Autodesk Inventor part; units mm, degrees
ref_plane "YZ Plane" through (0, 0, 0) normal (1, 0, 0) x (0, 1, 0)
ref_plane "XZ Plane" through (0, 0, 0) normal (0, 1, 0) x (-1, 0, 0)
ref_plane "XY Plane" through (0, 0, 0) normal (0, 0, 1) x (1, 0, 0)
sketch "Sketch1" plane through (0, 0, 0) normal (0, 0, 1) x (1, 0, 0)
  line L0 (0, 0) -> (125, 0)
  line L1 (125, 0) -> (125, 50)
  line L2 (125, 50) -> (0, 50)
  line L3 (0, 50) -> (0, 0)
  dimension "d0" = 125
  dimension "d1" = 50
extrude "Extrusion1" add sketch "Sketch1" along normal blind 6.731
sketch "Sketch4" plane through (0, 0, 0) normal (0, 0, -1) x (-1, 0, 0)
  line L0 (-125, 50) -> (0, 50)
  line L1 (-125, 0) -> (-125, 50)
  line L2 (-125, 4.3708) -> (-86.0388, 50)
  line L3 (-112.0129, 19.5805) -> (-106.8941, 15.2097)
  line L4 (-106.8941, 15.2097) -> (-93.907, 30.4195)
  line L5 (-93.907, 30.4195) -> (-99.0259, 34.7903)
  line L6 (0, 0) -> (-125, 0)
  line L7 (-125, 4.3708) -> (-119.8812, 0)
  circle A0 centre (-114.3237, 11.6915) radius 1.588
  dimension "d25" = 6.731
  dimension "d26" = 20
  dimension "d27" = 20
  dimension "d28" = 6.731
  dimension "d29" = 3.176
  dimension "d30" = 3.3655
  dimension "d31" = 7.5
  dimension "d40" = 60
extrude "LCD_Cut" cut sketch "Sketch4" against normal up to next contours L0 L2 L1 | L5 L4 L3 L2 | A0
sketch "Sketch2" plane through (0, 0, 6.731) normal (0, 0, 1) x (1, 0, 0)
  line L0 (0, 0) -> (125, 0)
  line L1 (125, 0) -> (125, 50)
  line L2 (0, 50) -> (0, 0)
  line L3 (20, 0) -> (40, 0)
  line L4 (40, 0) -> (40, -6.731)
  line L5 (40, -6.731) -> (20, -6.731)
  line L6 (20, -6.731) -> (20, 0)
  line L7 (105, 0) -> (85, 0)
  line L8 (85, 0) -> (85, -6.731)
  line L9 (85, -6.731) -> (105, -6.731)
  line L10 (105, -6.731) -> (105, 0)
  line L11 (0, 35) -> (-6.731, 35)
  line L12 (-6.731, 35) -> (-6.731, 15)
  line L13 (-6.731, 15) -> (0, 15)
  line L14 (0, 15) -> (0, 35)
  line L15 (86.0388, 50) -> (0, 50)
  line L16 (20, 50) -> (40, 50)
  line L17 (40, 50) -> (40, 56.731)
  line L18 (40, 56.731) -> (20, 56.731)
  line L19 (20, 56.731) -> (20, 50)
  point P0 (-6.731, 25)
  point P1 (0, 25)
  dimension "d4" = 6.731
  dimension "d5" = 20
  dimension "d6" = 20
  dimension "d7" = 20
extrude "Tabs Pos" add sketch "Sketch2" against normal blind 6.731
sketch "Sketch3" plane through (0, 0, 0) normal (0, 0, -1) x (-1, 0, 0)
  line L0 (0, 50) -> (0, 0)
  line L1 (-86.0388, 50) -> (0, 50)
  line L2 (-20, -6.731) -> (-20, 0)
  circle A0 centre (-50, 45) radius 1.588
  circle A1 centre (-10, 45) radius 1.588
  circle A2 centre (-10, 5) radius 1.588
  circle A3 centre (-50, 5) radius 1.588
  line L3 (-50, 45) -> (-50, 5) construction
  line L4 (-10, 45) -> (-50, 45) construction
  line L5 (-50, 5) -> (-10, 45) construction
  circle A4 centre (-30, 25) radius 23.75
  point P0 (-150, 55)
  dimension "d10" = 3.176
  dimension "d11" = 40
  dimension "d12" = 5
  dimension "d13" = 50
  dimension "d14" = 10
  dimension "d15" = 47.5
extrude "Fan" cut sketch "Sketch3" against normal up to next
equation "\"d2\" = THICKB"
equation "\"d25\" = THICKB"
equation "\"d28\" = THICKB"
equation "\"d30\" = 0.5 * THICKB"
equation "\"d4\" = THICKB"
equation "\"d8\" = THICKB"
equation "\"d12\" = -0.5 * d11 + 0.5 * d13"
equation "\"THICKA\" = 3.175"
equation "\"THICKB\" = 6.731"
equation "\"THICKC\" = 12.7"
equation "\"THICKPLY\" = 5"
equation "\"MAGDIA\" = 9.5"
equation "\"BALLDIA\" = 12"
properties part number "Controller_Side_A"
The listing builds one solid part. Answer for the finished solid, in the listing's coordinates (mm). A direction names the side the tool comes from. Give positions to 0.01 mm unless a question says otherwise; leave off trailing zeros. Write each loop counter-clockwise with the first axis right and the second up, starting at its lowest first coordinate (ties: lowest second). Pieces come first, ordered by that corner, then holes.
1) Section C-C (x = 50) is taken. Write down the section's boundary in (y, z).
2) Section A-A (x = 30) is taken. Write down the section's boundary in (y, z), and give its area (3 significant figures).
3) Given P1, Ø1, axis at x = 88, z = 2, coming from the +Y side; P2, Ø5, axis at x = 50, y = 45, coming from the +Z side; P3, Ø2, axis at y = -4, z = 2.5, coming from the +X side; P4, Ø2, axis at x = 54.5, z = 4, coming from the -Y side, each flat-ended and moving along its own axis, determine where each tip first touches the part or whether it passes through.
4) Section B-B (y = 25) is taken. Write down the section's boundary in (x, z), and give its area (3 significant figures).
5) For a pull along X with two mould halves and no side action, classify faces 1 (the face through (20, 53, 3)), 2 (the face through (40, 53, 3)), 3 (the face through (51.26, 4.034, 3.318)), 4 (the face through (51.17, 46.073, 3.318)) as pulls with the +X half, pulls with the -X half, needs draft (parallel to the pull), parting line crosses it, or undercut.
6) A tool of negligible diameter and unlimited length cuts with its end or side. For faces 5 (the face through (100.5, 22.7, 3.3)), 6 (the face through (30, 56.731, 3)), 7 (the face through (115, 0, 3)), 8 (the face through (10, 50, 3)), 9 (the face through (-3, 15, 3)), from which of +Z, -Z, +X, -X, +Y, -Y can it reach the whole face along a straight path? Write none if from no direction.
7) Find the intervals of material crossed by L1, parallel to Y at x = 30, z = 4; L2, parallel to Y at x = 10, z = 4.5; L3, parallel to X at y = -2, z = 2.25, in increasing order.
8) Section D-D (y = 45) is taken. Write down the section's boundary in (x, z).
Response:
1. outline: (0, 0) - (3.41, 0) - (3.41, 6.73) - (0, 6.73) - close; (6.59, 0) - (12.19, 0) - (12.19, 6.73) - (6.59, 6.73) - close; (37.81, 0) - (43.41, 0) - (43.41, 6.73) - (37.81, 6.73) - close; (46.59, 0) - (50, 0) - (50, 6.73) - (46.59, 6.73) - close
2. outline: (-6.73, 0) - (1.25, 0) - (1.25, 6.73) - (-6.73, 6.73) - close; (48.75, 0) - (56.73, 0) - (56.73, 6.73) - (48.75, 6.73) - close
2. area: 107 mm2
3. P1: stops at y = 48.29
3. P2: stops at z = 6.73
3. P3: stops at x = 105
3. P4: stops at y = 0
4. outline: (-6.73, 0) - (6.25, 0) - (6.25, 6.73) - (-6.73, 6.73) - close; (53.75, 0) - (98.53, 0) - (98.53, 6.73) - (53.75, 6.73) - close
4. area: 389 mm2
5. face 1: pulls with the -X half
5. face 2: pulls with the +X half
5. face 3: undercut
5. face 4: undercut
6. face 5: +Z, -Z
6. face 6: +Z, -Z, +X, -X, +Y
6. face 7: +Z, -Z, +X, -Y
6. face 8: +Z, -Z, -X, +Y
6. face 9: +Z, -Z, -X, -Y
7. L1: y = -6.73 to 1.25, 48.75 to 56.73
7. L2: y = 0 to 3.41, 6.59 to 12.19, 37.81 to 43.41, 46.59 to 50
7. L3: x = 20 to 40, 85 to 105
8. outline: (0, 0) - (8.41, 0) - (8.41, 6.73) - (0, 6.73) - close; (11.59, 0) - (17.19, 0) - (17.19, 6.73) - (11.59, 6.73) - close; (42.81, 0) - (48.41, 0) - (48.41, 6.73) - (42.81, 6.73) - close; (51.59, 0) - (90.31, 0) - (90.31, 6.73) - (51.59, 6.73) - close
